Source: CAD feature listing. Evaluate the final solid. Frame: model axes, mm. Face numbers are marked on the shaded views. Round coordinates to 2 decimals unless told otherwise and drop trailing zeros. Loops run counter-clockwise (first coordinate to the right, second up) from the corner with the lowest first, then second, coordinate; pieces in that order, holes last. Notation, with made-up numbers: (-25.75, -10) -> (17.25, -10) arc R31 ccw to (17.25, 25) -> close; hole circle Ø8 at (34, 51). An arc over 180 degrees is marked (long way). Put each result on its own line as item: value. Start each with the question number.
1. Cut plane A-A (x = 0). Return the cut outline in (y, z).
2. Cut plane C-C (y = -10.75). Return the cut outline in (x, z), then the cut area to 3 significant figures.
3. Draft query along Z for the marked faces 1, 2 and 3. Return one class per face: pulls with the +Z half, pulls with the -Z half, needs draft (parallel to the pull), parting line crosses it, or undercut.
4. Material intervals for L1, parallel to Z at x = 0, y = -2.6; L2, parallel to Y at x = -4.5, z = -0.5; L3, parallel to Z at x = -1, y = -2.75, sorted ascending.
5. Cut plane B-B (y = -2.5). Return the cut outline in (x, z), then the cut area to 3 significant figures.
6. Contact query for flat-ended pins moving along their axis: pin 1 (3 mm diameter, centred on x = 6.5, z = 7, fed in from -Y); pin 2 (8 mm diameter, centred on x = 1, y = -7.5, fed in from +Z); pin 3 (2 mm diameter, centred on x = 7.5, z = -9, fed in from +Y). Output: stop coordinate, or through.
```python
from build123d import *

# Parameters (mm, degrees)
F0_R     = 1.5
F1_DEPTH = 15
F2_DEPTH = 4
F3_R     = 2.5
F4_DEPTH = 25
F5_R     = 1


with BuildPart() as f1:
    # F0 (on Front) → F1 (new body)
    with BuildSketch(Plane.XZ):
        with Locations((0, -10.47795)):
            Circle(F0_R)
    extrude(amount=F1_DEPTH)

    # F0 (on Front) → F2 (join)
    with BuildSketch(Plane.XZ):
        with BuildLine():
            Line((-11.9213, 9.103989), (-5.846707, -13.813617))
            ThreePointArc((-5.846707, -13.813617), (0, -15), (5.846707, -13.813617))
            Line((5.846707, -13.813617), (11.9213, 9.103989))
            ThreePointArc((11.9213, 9.103989), (0, 15), (-11.9213, 9.103989))
        make_face()
        with Locations((0, -10.47795)):
            Circle(F0_R, mode=Mode.SUBTRACT)
    extrude(amount=F2_DEPTH)

    # F3 (on face) → F4 (cut)
    with BuildSketch(Plane(origin=(0, 0, 0), x_dir=(-1, 0, 0), z_dir=(0, 1, 0))):
        Circle(F3_R)
    extrude(amount=-F4_DEPTH, mode=Mode.SUBTRACT)

    # F5
    f5_edges = [f1.edges().sort_by_distance(p)[0] for p in [
        (0, -4, 15),
        (11.9213, -2, 9.103989),
        (-11.9213, -2, 9.103989),
        (0, 0, 15),
        (5.846707, -2, -13.813617),
        (0, -4, -15),
        (0, 0, -15),
        (-5.846707, -2, -13.813617),
        (-8.884003, 0, -2.354814),
        (-8.884003, -4, -2.354814),
        (8.884003, -4, -2.354814),
        (8.884003, 0, -2.354814),
    ]]
    fillet(f5_edges, radius=F5_R)


solid = f1.part
```
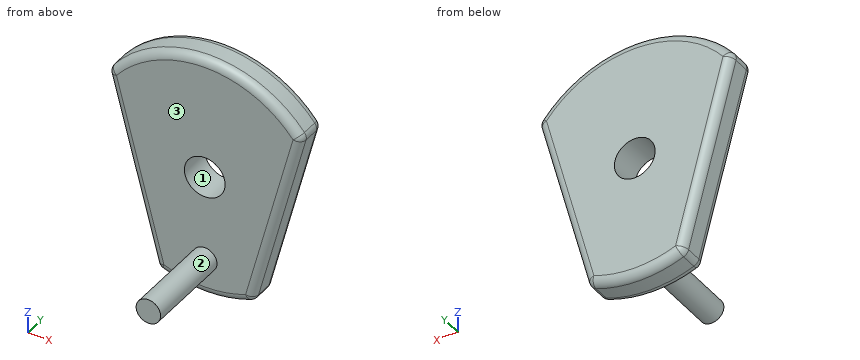
Solution:
1. outline: (-15, -11.98) -> (-4, -11.98) -> (-4, -14) arc R1 ccw to (-3, -15) -> (-1, -15) arc R1 ccw to (0, -14) -> (0, -2.5) -> (-4, -2.5) -> (-4, -8.98) -> (-15, -8.98) -> close; (-4, 2.5) -> (0, 2.5) -> (0, 14) arc R1 ccw to (-1, 15) -> (-3, 15) arc R1 ccw to (-4, 14) -> close
2. outline: circle Ø3 at (0, -10.48)
2. area: 7.07 mm^2
3. face 1: undercut
3. face 2: parting line crosses it
3. face 3: needs draft
4. L1: z = -15 to -2.5, 2.5 to 15
4. L2: y = -4 to 0
4. L3: z = -14.97 to -2.29, 2.29 to 14.97
5. outline: (-11.79, 8.62) -> (-5.97, -13.33) arc R1 ccw to (-5.37, -14.01) arc R15 ccw to (5.37, -14.01) arc R1 ccw to (5.97, -13.33) -> (11.79, 8.62) arc R1 ccw to (11.6, 9.51) arc R15 ccw to (-11.6, 9.51) arc R1 ccw to start; hole circle Ø5 at (0, 0)
5. area: 495 mm^2
6. pin 1: stops at y = -4
6. pin 2: stops at z = 14.84
6. pin 3: stops at y = -0.07
